from build123d import *

# Parameters (mm, degrees)
EXTRUDE_1_DEPTH     = 10
FILLET_3_R          = 0.3
SKETCH_2_R          = 2
CUT_EXTRUDE_1_DEPTH = 6


with BuildPart() as part:
    # 草图1 → 凸台-拉伸1 (new body)
    with BuildSketch(Plane.XY):
        with BuildLine():
            Line((-3, 4.3), (3, 4.3))
            Line((3, 4.3), (3, 3.8))
            ThreePointArc((3, 3.8), (3.146446609, 3.446446609), (3.5, 3.3))
            Line((3.5, 3.3), (5.1, 3.3))
            Line((5.1, 3.3), (5.1, 3.128427125))
            ThreePointArc((5.1, 3.128427125), (4.947759065, 2.36306026), (4.514213562, 1.714213562))
            Line((4.514213562, 1.714213562), (3.385786438, 0.585786438))
            ThreePointArc((3.385786438, 0.585786438), (2.73693974, 0.152240935), (1.971572875, 0))
            Line((1.971572875, 0), (-1.971572875, 0))
            ThreePointArc((-1.971572875, 0), (-2.73693974, 0.152240935), (-3.385786438, 0.585786438))
            Line((-3.385786438, 0.585786438), (-4.514213562, 1.714213562))
            ThreePointArc((-4.514213562, 1.714213562), (-4.947759065, 2.36306026), (-5.1, 3.128427125))
            Line((-5.1, 3.128427125), (-5.1, 3.3))
            Line((-5.1, 3.3), (-3.5, 3.3))
            ThreePointArc((-3.5, 3.3), (-3.146446609, 3.446446609), (-3, 3.8))
            Line((-3, 3.8), (-3, 4.3))
        make_face()
    extrude(amount=EXTRUDE_1_DEPTH)

    # 圆角3
    # the kernel refuses this fillet: 0.3 mm, written as the material it takes off along each edge
    with BuildSketch(Plane(origin=(-3, 3.8, 10), x_dir=(0, 0, -1), z_dir=(0, 1, 0)), Plane(origin=(3, 5.05, 10), x_dir=(0, 0, -1), z_dir=(0, -1, 0))) as fillet_3_piece_1:
        with BuildLine():
            CenterArc((FILLET_3_R, -FILLET_3_R), FILLET_3_R, 90, 90)
            Line((0, -FILLET_3_R), (0, 0))
            Line((0, 0), (FILLET_3_R, 0))
        make_face()
    extrude(amount=1.25, mode=Mode.SUBTRACT)
    with BuildSketch(Plane(origin=(3, 5.05, 0), x_dir=(0, 0, 1), z_dir=(0, -1, 0)), Plane(origin=(-3, 3.8, 0), x_dir=(0, 0, 1), z_dir=(0, 1, 0))) as fillet_3_piece_2:
        with BuildLine():
            CenterArc((FILLET_3_R, FILLET_3_R), FILLET_3_R, 180, 90)
            Line((0, FILLET_3_R), (0, 0))
            Line((0, 0), (FILLET_3_R, 0))
        make_face()
    extrude(amount=1.25, mode=Mode.SUBTRACT)
    with BuildSketch(Plane(origin=(4.514213562, 1.714213562, 10), x_dir=(0, 0, -1), z_dir=(-0.7071067811865436, -0.7071067811865515, 0)), Plane(origin=(-3.385786438, 0.585786438, 10), x_dir=(0, 0, -1), z_dir=(-0.7071067811865436, 0.7071067811865515, 0))) as fillet_3_piece_3:
        with BuildLine():
            CenterArc((FILLET_3_R, -FILLET_3_R), FILLET_3_R, 90, 90)
            Line((0, -FILLET_3_R), (0, 0))
            Line((0, 0), (FILLET_3_R, 0))
        make_face()
    extrude(amount=1.595836944, mode=Mode.SUBTRACT)
    with BuildSketch(Plane(origin=(1.971572875, 2, 10), x_dir=(0.7071067811865542, -0.7071067811865409, 0), z_dir=(0.7071067811865409, 0.7071067811865542, 0))) as fillet_3_piece_4:
        with BuildLine():
            CenterArc((2 - FILLET_3_R, FILLET_3_R), FILLET_3_R, 270, 90)
            Line((2 - FILLET_3_R, 0), (2, 0))
            Line((2, 0), (2, FILLET_3_R))
        make_face()
    revolve(axis=Axis((1.971572875, 2, 10), (0, 0, -1)), revolution_arc=45, mode=Mode.SUBTRACT)
    with BuildSketch(Plane(origin=(1.971572875, 0, 10), x_dir=(0, 0, -1), z_dir=(-1, 0, 0))) as fillet_3_piece_5:
        with BuildLine():
            CenterArc((FILLET_3_R, -FILLET_3_R), FILLET_3_R, 90, 90)
            Line((0, -FILLET_3_R), (0, 0))
            Line((0, 0), (FILLET_3_R, 0))
        make_face()
    extrude(amount=3.943145751, mode=Mode.SUBTRACT)
    with BuildSketch(Plane(origin=(-1.971572875, 2, 10), x_dir=(0, -1, 0), z_dir=(1, 0, 0))) as fillet_3_piece_6:
        with BuildLine():
            CenterArc((2 - FILLET_3_R, FILLET_3_R), FILLET_3_R, 270, 90)
            Line((2 - FILLET_3_R, 0), (2, 0))
            Line((2, 0), (2, FILLET_3_R))
        make_face()
    revolve(axis=Axis((-1.971572875, 2, 10), (0, 0, -1)), revolution_arc=45, mode=Mode.SUBTRACT)
    with BuildSketch(Plane(origin=(-3.1, 3.128427125, 10), x_dir=(-0.7071067811865485, -0.7071067811865466, 0), z_dir=(0.7071067811865466, -0.7071067811865485, 0))) as fillet_3_piece_7:
        with BuildLine():
            CenterArc((2 - FILLET_3_R, FILLET_3_R), FILLET_3_R, 270, 90)
            Line((2 - FILLET_3_R, 0), (2, 0))
            Line((2, 0), (2, FILLET_3_R))
        make_face()
    revolve(axis=Axis((-3.1, 3.128427125, 10), (0, 0, -1)), revolution_arc=45, mode=Mode.SUBTRACT)
    with BuildSketch(Plane(origin=(-5.85, 3.3, 10), x_dir=(0, 0, -1), z_dir=(1, 0, 0)), Plane(origin=(3.5, 3.3, 10), x_dir=(0, 0, -1), z_dir=(1, 0, 0))) as fillet_3_piece_8:
        with BuildLine():
            CenterArc((FILLET_3_R, -FILLET_3_R), FILLET_3_R, 90, 90)
            Line((0, -FILLET_3_R), (0, 0))
            Line((0, 0), (FILLET_3_R, 0))
        make_face()
    extrude(amount=2.35, mode=Mode.SUBTRACT)
    with BuildSketch(Plane(origin=(-3.5, 3.8, 10), x_dir=(0, -1, 0), z_dir=(-1, 0, 0))) as fillet_3_piece_9:
        with BuildLine():
            CenterArc((0.5 + FILLET_3_R, -FILLET_3_R), FILLET_3_R, 90, 90)
            Line((0.5 + FILLET_3_R, 0), (0.5, 0))
            Line((0.5, 0), (0.5, -FILLET_3_R))
        make_face()
    revolve(axis=Axis((-3.5, 3.8, 10), (0, 0, 1)), revolution_arc=90, mode=Mode.SUBTRACT)
    with BuildSketch(Plane(origin=(3.5, 3.3, 0), x_dir=(0, 0, 1), z_dir=(1, 0, 0)), Plane(origin=(-5.85, 3.3, 0), x_dir=(0, 0, 1), z_dir=(1, 0, 0))) as fillet_3_piece_10:
        with BuildLine():
            CenterArc((FILLET_3_R, FILLET_3_R), FILLET_3_R, 180, 90)
            Line((0, FILLET_3_R), (0, 0))
            Line((0, 0), (FILLET_3_R, 0))
        make_face()
    extrude(amount=2.35, mode=Mode.SUBTRACT)
    with BuildSketch(Plane(origin=(3.5, 3.8, 0), x_dir=(-1, 0, 0), z_dir=(0, 1, 0))) as fillet_3_piece_11:
        with BuildLine():
            CenterArc((0.5 + FILLET_3_R, FILLET_3_R), FILLET_3_R, 180, 90)
            Line((0.5 + FILLET_3_R, 0), (0.5, 0))
            Line((0.5, 0), (0.5, FILLET_3_R))
        make_face()
    revolve(axis=Axis((3.5, 3.8, 0), (0, 0, 1)), revolution_arc=90, mode=Mode.SUBTRACT)
    with BuildSketch(Plane(origin=(-3.385786438, 0.585786438, 0), x_dir=(0, 0, 1), z_dir=(-0.7071067811865436, 0.7071067811865515, 0)), Plane(origin=(4.514213562, 1.714213562, 0), x_dir=(0, 0, 1), z_dir=(-0.7071067811865436, -0.7071067811865515, 0))) as fillet_3_piece_12:
        with BuildLine():
            CenterArc((FILLET_3_R, FILLET_3_R), FILLET_3_R, 180, 90)
            Line((0, FILLET_3_R), (0, 0))
            Line((0, 0), (FILLET_3_R, 0))
        make_face()
    extrude(amount=1.595836944, mode=Mode.SUBTRACT)
    with BuildSketch(Plane(origin=(-1.971572875, 2, 0), x_dir=(0, -1, 0), z_dir=(1, 0, 0))) as fillet_3_piece_13:
        with BuildLine():
            CenterArc((2 - FILLET_3_R, -FILLET_3_R), FILLET_3_R, 0, 90)
            Line((2 - FILLET_3_R, 0), (2, 0))
            Line((2, 0), (2, -FILLET_3_R))
        make_face()
    revolve(axis=Axis((-1.971572875, 2, 0), (0, 0, -1)), revolution_arc=45, mode=Mode.SUBTRACT)
    with BuildSketch(Plane(origin=(1.971572875, 0, 0), x_dir=(0, 0, 1), z_dir=(-1, 0, 0))) as fillet_3_piece_14:
        with BuildLine():
            CenterArc((FILLET_3_R, FILLET_3_R), FILLET_3_R, 180, 90)
            Line((0, FILLET_3_R), (0, 0))
            Line((0, 0), (FILLET_3_R, 0))
        make_face()
    extrude(amount=3.943145751, mode=Mode.SUBTRACT)
    with BuildSketch(Plane(origin=(1.971572875, 2, 0), x_dir=(0.7071067811865542, -0.7071067811865409, 0), z_dir=(0.7071067811865409, 0.7071067811865542, 0))) as fillet_3_piece_15:
        with BuildLine():
            CenterArc((2 - FILLET_3_R, -FILLET_3_R), FILLET_3_R, 0, 90)
            Line((2 - FILLET_3_R, 0), (2, 0))
            Line((2, 0), (2, -FILLET_3_R))
        make_face()
    revolve(axis=Axis((1.971572875, 2, 0), (0, 0, -1)), revolution_arc=45, mode=Mode.SUBTRACT)
    with BuildSketch(Plane(origin=(3.1, 3.128427125, 0), x_dir=(1, 0, 0), z_dir=(0, 1, 0))) as fillet_3_piece_16:
        with BuildLine():
            CenterArc((2 - FILLET_3_R, -FILLET_3_R), FILLET_3_R, 0, 90)
            Line((2 - FILLET_3_R, 0), (2, 0))
            Line((2, 0), (2, -FILLET_3_R))
        make_face()
    revolve(axis=Axis((3.1, 3.128427125, 0), (0, 0, -1)), revolution_arc=45, mode=Mode.SUBTRACT)
    with BuildSketch(Plane(origin=(3.1, 3.128427125, 10), x_dir=(1, 0, 0), z_dir=(0, 1, 0))) as fillet_3_piece_17:
        with BuildLine():
            CenterArc((2 - FILLET_3_R, FILLET_3_R), FILLET_3_R, 270, 90)
            Line((2 - FILLET_3_R, 0), (2, 0))
            Line((2, 0), (2, FILLET_3_R))
        make_face()
    revolve(axis=Axis((3.1, 3.128427125, 10), (0, 0, -1)), revolution_arc=45, mode=Mode.SUBTRACT)
    with BuildSketch(Plane(origin=(-3.1, 3.128427125, 0), x_dir=(-0.7071067811865485, -0.7071067811865466, 0), z_dir=(0.7071067811865466, -0.7071067811865485, 0))) as fillet_3_piece_18:
        with BuildLine():
            CenterArc((2 - FILLET_3_R, -FILLET_3_R), FILLET_3_R, 0, 90)
            Line((2 - FILLET_3_R, 0), (2, 0))
            Line((2, 0), (2, -FILLET_3_R))
        make_face()
    revolve(axis=Axis((-3.1, 3.128427125, 0), (0, 0, -1)), revolution_arc=45, mode=Mode.SUBTRACT)
    with BuildSketch(Plane(origin=(3.5, 3.8, 10), x_dir=(-1, 0, 0), z_dir=(0, 1, 0))) as fillet_3_piece_19:
        with BuildLine():
            CenterArc((0.5 + FILLET_3_R, -FILLET_3_R), FILLET_3_R, 90, 90)
            Line((0.5 + FILLET_3_R, 0), (0.5, 0))
            Line((0.5, 0), (0.5, -FILLET_3_R))
        make_face()
    revolve(axis=Axis((3.5, 3.8, 10), (0, 0, 1)), revolution_arc=90, mode=Mode.SUBTRACT)
    with BuildSketch(Plane(origin=(-3.5, 3.8, 0), x_dir=(0, -1, 0), z_dir=(-1, 0, 0))) as fillet_3_piece_20:
        with BuildLine():
            CenterArc((0.5 + FILLET_3_R, FILLET_3_R), FILLET_3_R, 180, 90)
            Line((0.5 + FILLET_3_R, 0), (0.5, 0))
            Line((0.5, 0), (0.5, FILLET_3_R))
        make_face()
    revolve(axis=Axis((-3.5, 3.8, 0), (0, 0, 1)), revolution_arc=90, mode=Mode.SUBTRACT)
    with BuildSketch(Plane(origin=(-5.1, 3.128427125, 0), x_dir=(0, 0, 1), z_dir=(0, 1, 0)), Plane(origin=(5.1, 4.05, 0), x_dir=(0, 0, 1), z_dir=(0, -1, 0))) as fillet_3_piece_21:
        with BuildLine():
            CenterArc((FILLET_3_R, FILLET_3_R), FILLET_3_R, 180, 90)
            Line((0, FILLET_3_R), (0, 0))
            Line((0, 0), (FILLET_3_R, 0))
        make_face()
    extrude(amount=0.921572875, mode=Mode.SUBTRACT)
    with BuildSketch(Plane(origin=(5.1, 4.05, 10), x_dir=(0, 0, -1), z_dir=(0, -1, 0)), Plane(origin=(-5.1, 3.128427125, 10), x_dir=(0, 0, -1), z_dir=(0, 1, 0))) as fillet_3_piece_22:
        with BuildLine():
            CenterArc((FILLET_3_R, -FILLET_3_R), FILLET_3_R, 90, 90)
            Line((0, -FILLET_3_R), (0, 0))
            Line((0, 0), (FILLET_3_R, 0))
        make_face()
    extrude(amount=0.921572875, mode=Mode.SUBTRACT)

    # 草图2 → 切除-拉伸1 (cut)
    with BuildSketch(Plane(origin=(0, 4.3, 0), x_dir=(1, 0, 0), z_dir=(0, 1, 0))):
        with Locations(Location((0, -3, 0), (0, 0, 270))):
            Circle(SKETCH_2_R)
    extrude(amount=-CUT_EXTRUDE_1_DEPTH, mode=Mode.SUBTRACT)


solid = part.part
Could you check a few things on this model? Use its own coordinates, in mm. A direction names the side the tool comes from. Give positions to 0.01 mm unless a question says otherwise; leave off trailing zeros. Order: outer loops, then holes, each group sorted by start corner. A loop starts at its lowest first (then second) coordinate and runs counter-clockwise, first axis right, second up. Notation, with made-up numbers: (21, 58) -> (60, 58) arc R12 cw to (60, 80) -> close; hole circle Ø9 at (15.25, 72.25). An arc over 180 degrees is marked (long way). Return JSON: item names as keys, results as strings.
1. Thinking about a two-plate mould opening in X: for faces 3 (the cylindrical face through (-3.878, 1.206, 0.086)), 4 (the flat face through (4, 3.3, 5)), 5 (the cylindrical face through (-2, 2, 3)), 6 (the cylindrical face through (2.747, 0.156, 4.934)), which applies, pulls with the +X half, pulls with the -X half, needs draft (parallel to the pull), parting line crosses it, or undercut?
Answer list:
{"face 3": "pulls with the -X half", "face 4": "needs draft", "face 5": "undercut", "face 6": "pulls with the +X half"}
2. Imagine slicing it at A-A on x = 0. List the corners of the cut face in (y, z) for me, then the cut area to 3 significant figures.
Answer list:
{"outline": "(0, 0.3) arc R0.3 ccw to (0.3, 0) -> (4.3, 0) -> (4.3, 1) -> (0, 1) -> close; (0, 5) -> (4.3, 5) -> (4.3, 10) -> (0.3, 10) arc R0.3 ccw to (0, 9.7) -> close", "area": "25.8 mm2"}
3. I need wall thicknesses on line 1 (X direction, y = 1.35, z = 4.5); line 2 (X direction, y = 1.35, z = 2); line 3 (Z direction, x = 4.5, y = 3.2). Which ranges of each line are inside material? Lowest first, please. Write a range as from..to.
Answer list:
{"line 1": "x = -4.15..-1.32, 1.32..4.15", "line 2": "x = -4.15..-1.73, 1.73..4.15", "line 3": "z = 0.08..9.92"}
4. For pin 1 Ø0.8 at (x, z) = (-4, 4) entering from +Y; pin 2 Ø0.6 at (y, z) = (4, 6) entering from -X; pin 3 Ø1.5 at (y, z) = (2, 1.5) entering from -X, each with a flat end and sliding along its axis, tell me the tip position at first contact or that it passes through.
Answer list:
{"pin 1": "stops at y = 3.3", "pin 2": "stops at x = -3.01", "pin 3": "stops at x = -5.06"}
5. Imagine slicing it at C-C on z = 3. List the corners of the cut face in (x, y) for me, then the cut area to 3 significant figures.
Answer list:
{"outline": "(-5.1, 3.13) arc R2 ccw to (-4.51, 1.71) -> (-3.39, 0.59) arc R2 ccw to (-2, 0) -> (-2, 4.3) -> (-3, 4.3) -> (-3, 3.8) arc R0.5 cw to (-3.5, 3.3) -> (-5.1, 3.3) -> close; (2, 0) arc R2 ccw to (3.39, 0.59) -> (4.51, 1.71) arc R2 ccw to (5.1, 3.13) -> (5.1, 3.3) -> (3.5, 3.3) arc R0.5 cw to (3, 3.8) -> (3, 4.3) -> (2, 4.3) -> close", "area": "16.9 mm2"}
6. On a 3-axis mill with a long thin cutter (end or side, diameter ignored), from which of +Z, -Z, +X, -X, +Y, -Y can I reach the whole of each face in a straight line? I mean faces 1 (the flat face through (-4, 3.3, 5)), 2 (the flat face through (0, 4.3, 6)). Say none if no direction works.
Answer list:
{"face 1": "+Z, -Z, -X, +Y", "face 2": "+Z, -Z, +X, -X, +Y"}
7. Imagine slicing it at B-B on z = 6.5. List the corners of the cut face in (x, y) for me, then the cut area to 3 significant figures.
Answer list:
{"outline": "(-5.1, 3.13) arc R2 ccw to (-4.51, 1.71) -> (-3.39, 0.59) arc R2 ccw to (-1.97, 0) -> (1.97, 0) arc R2 ccw to (3.39, 0.59) -> (4.51, 1.71) arc R2 ccw to (5.1, 3.13) -> (5.1, 3.3) -> (3.5, 3.3) arc R0.5 cw to (3, 3.8) -> (3, 4.3) -> (-3, 4.3) -> (-3, 3.8) arc R0.5 cw to (-3.5, 3.3) -> (-5.1, 3.3) -> close", "area": "34.1 mm2"}
8. Imagine slicing it at D-D on x = 1.25. List the corners of the cut face in (y, z) for me.
Answer list:
{"outline": "(0, 0.3) arc R0.3 ccw to (0.3, 0) -> (4.3, 0) -> (4.3, 1.44) -> (0, 1.44) -> close; (0, 4.56) -> (4.3, 4.56) -> (4.3, 10) -> (0.3, 10) arc R0.3 ccw to (0, 9.7) -> close"}
